```python
from build123d import *

# Parameters (mm, degrees)
SKETCH1_W            = 23
SKETCH1_H            = 12
BOSS_EXTRUDE1_DEPTH  = 18
SKETCH2_W            = 32
SKETCH2_H            = 12
BOSS_EXTRUDE2_DEPTH  = 2.5
SKETCH3_W            = 23
SKETCH3_H            = 12
BOSS_EXTRUDE3_DEPTH  = 4
BOSS_EXTRUDE4_DEPTH  = 4.5
FILLET1_R            = 1
FILLET2_R            = 0.5
CUT_EXTRUDE2_DEPTH   = 21.5
SKETCH5_R            = 2.5
BOSS_EXTRUDE5_DEPTH  = 3
SKETCH6_R            = 1
CUT_EXTRUDE1_DEPTH   = 3
BOSS_EXTRUDE11_DEPTH = 2
FILLET3_R            = 0.5


with BuildPart() as part:
    # Sketch1 → Boss-Extrude1 (new body)
    with BuildSketch(Plane(origin=(0, 0, 0), x_dir=(1, 0, 0), z_dir=(0, 1, 0))):
        Rectangle(SKETCH1_W, SKETCH1_H)
    extrude(amount=BOSS_EXTRUDE1_DEPTH)

    # Sketch2 → Boss-Extrude2 (add)
    with BuildSketch(Plane(origin=(0, 18, 0), x_dir=(1, 0, 0), z_dir=(0, 1, 0))):
        Rectangle(SKETCH2_W, SKETCH2_H)
    extrude(amount=BOSS_EXTRUDE2_DEPTH)

    # Sketch3 → Boss-Extrude3 (add)
    with BuildSketch(Plane(origin=(0, 20.5, 0), x_dir=(1, 0, 0), z_dir=(0, 1, 0))):
        Rectangle(SKETCH3_W, SKETCH3_H)
    extrude(amount=BOSS_EXTRUDE3_DEPTH)

    # Sketch4 → Boss-Extrude4 (add)
    with BuildSketch(Plane(origin=(0, 24.5, 0), x_dir=(1, 0, 0), z_dir=(0, 1, 0))):
        with BuildLine():
            Line((-0.802804538, 3), (0.303847577, 3))
            ThreePointArc((0.303847577, 3), (11.5, 0), (0.303847577, -3))
            Line((0.303847577, -3), (-0.802804538, -3))
            ThreePointArc((-0.802804538, -3), (-3.802804538, 0), (-0.802804538, 3))
        make_face()
    extrude(amount=BOSS_EXTRUDE4_DEPTH)

    # Fillet1
    fillet1_edges = [part.edges().sort_by_distance(p)[0] for p in [
        (11.5, 22.5, 6),
        (11.5, 22.5, -6),
        (-11.5, 22.5, -6),
        (-11.5, 22.5, 6),
        (11.5, 9, 6),
        (-11.5, 9, 6),
        (-11.5, 9, -6),
        (11.5, 9, -6),
    ]]
    fillet(fillet1_edges, radius=FILLET1_R)

    # Fillet2
    fillet2_edges = [part.edges().sort_by_distance(p)[0] for p in [
        (16, 19.25, 6),
        (16, 19.25, -6),
        (-16, 19.25, -6),
        (-16, 19.25, 6),
    ]]
    fillet(fillet2_edges, radius=FILLET2_R)

    # Sketch7 → Cut-Extrude2 (cut, through all)
    with BuildSketch(Plane(origin=(0, 20.5, 0), x_dir=(1, 0, 0), z_dir=(0, 1, 0))):
        with BuildLine():
            Line((14.420576737, 0.3), (16, 0.3))
            Line((16, 0.3), (16, -0.3))
            Line((16, -0.3), (14.420576737, -0.3))
            ThreePointArc((14.420576737, -0.3), (12.53177403, 0), (14.420576737, 0.3))
        make_face()
    cut_extrude2 = extrude(amount=-CUT_EXTRUDE2_DEPTH, mode=Mode.SUBTRACT)

    # Mirror1: Cut-Extrude2 across plane
    add(cut_extrude2.mirror(Plane(origin=(0, 0, 0), x_dir=(0, 0, 1), z_dir=(1, 0, 0))), mode=Mode.SUBTRACT)

    # Sketch5 → Boss-Extrude5 (add)
    with BuildSketch(Plane(origin=(0, 29, 0), x_dir=(1, 0, 0), z_dir=(0, 1, 0))):
        with Locations((5.5, 0)):
            Circle(SKETCH5_R)
    extrude(amount=BOSS_EXTRUDE5_DEPTH)

    # Sketch6 → Cut-Extrude1 (cut)
    with BuildSketch(Plane(origin=(0, 32, 0), x_dir=(1, 0, 0), z_dir=(0, 1, 0))):
        with Locations((5.5, 0)):
            Circle(SKETCH6_R)
    extrude(amount=-CUT_EXTRUDE1_DEPTH, mode=Mode.SUBTRACT)

    # Sketch8 → Boss-Extrude11 (add)
    with BuildSketch(Plane(origin=(11.5, 0, 0), x_dir=(0, 0, -1), z_dir=(1, 0, 0))):
        with BuildLine():
            Line((-0.539222972, 6.176789317), (-0.474627778, 6.176789317))
            ThreePointArc((-0.474627778, 6.176789317), (-0.006925375, 6.5), (0.460777028, 6.176789317))
            Line((0.460777028, 6.176789317), (0.525372222, 6.176789317))
            ThreePointArc((0.525372222, 6.176789317), (1.493074625, 6), (0.525372222, 5.823210683))
            Line((0.525372222, 5.823210683), (0.460777028, 5.823210683))
            ThreePointArc((0.460777028, 5.823210683), (-0.006925375, 5.5), (-0.474627778, 5.823210683))
            Line((-0.474627778, 5.823210683), (-0.539222972, 5.823210683))
            ThreePointArc((-0.539222972, 5.823210683), (-1.506925375, 6), (-0.539222972, 6.176789317))
        make_face()
    extrude(amount=BOSS_EXTRUDE11_DEPTH)

    # Fillet3
    fillet3_edges = [part.edges().sort_by_distance(p)[0] for p in [
        (-3.802804538, 29, 0),
        (-0.249478481, 29, 3),
        (11.5, 29, 0),
        (-0.249478481, 29, -3),
    ]]
    fillet(fillet3_edges, radius=FILLET3_R)


solid = part.part
```
Could you check a few things on this model? Use its own coordinates, in mm. A direction names the side the tool comes from. Give positions to 0.01 mm unless a question says otherwise; leave off trailing zeros. Loops run counter-clockwise (first coordinate to the right, second up) from the corner with the lowest first, then second, coordinate; pieces in that order, holes last. Notation, with made-up numbers: (36, 73) -> (58, 73) arc R20 cw to (58, 84) -> close; hole circle Ø5 at (-21, 35). An arc over 180 degrees is marked (long way). Put each result on its own line as item: value.
(1) Imagine slicing it at C-C on x = -8. Write out the boundary of the cut face in (y, z).
Computed:
outline: (0, -6) -> (24.5, -6) -> (24.5, 6) -> (0, 6) -> close
(2) For faces 5 (the face through (11.5, 22, 0)), 6 (the face through (10, 24.5, -5)), 7 (the face through (-11.215, 22.528, -5.699)), which set-ups out of +Z, -Z, +X, -X, +Y, -Y let a thin tool reach every point of the face, with its end or its side?
Computed:
face 5: +Z, -Z, +X, +Y
face 6: -Z, +X, +Y
face 7: -Z, -X, +Y
(3) Imagine slicing it at B-B on y = 7. Write out the boundary of the cut face in (x, z), plus the area to 3 significant figures.
Computed:
outline: (-11.5, -5) arc R1 ccw to (-10.5, -6) -> (10.5, -6) arc R1 ccw to (11.5, -5) -> (11.5, 5) arc R1 ccw to (10.5, 6) -> (-10.5, 6) arc R1 ccw to (-11.5, 5) -> close
area: 275 mm^2
(4) Imagine slicing it at A-A on x = -13.5. Write out the boundary of the cut face in (y, z), plus the area to 3 significant figures.
Computed:
outline: (18, -6) -> (20.5, -6) -> (20.5, -0.97) -> (18, -0.97) -> close; (18, 0.97) -> (20.5, 0.97) -> (20.5, 6) -> (18, 6) -> close
area: 25.2 mm^2
(5) Please list where these lines run through material, in increasing order: probe 1 along Z at (x, y) = (-13.5, 19.2); probe 2 along X at (y, z) = (30.3, 0); probe 3 along X at (y, z) = (18.7, 0). Write a range as [from, to].
Computed:
probe 1: [-6, -0.97], [0.97, 6]
probe 2: [3, 4.5], [6.5, 8]
probe 3: [-12.53, 12.53]
(6) Thinking about a two-plate mould opening in X: for faces 1 (the face through (-11.5, 9, 0)), 2 (the face through (-15, 19, -0.3)), 3 (the face through (-12.533, 19.268, 0.038)), 4 (the face through (5, 29, 0)), which applies, pulls with the +X half, pulls with the -X half, needs draft (parallel to the pull), parting line crosses it, or undercut?
Computed:
face 1: pulls with the -X half
face 2: needs draft
face 3: undercut
face 4: undercut
(7) I'm going to push flat-ended pins straight in: pin 1 Ø3 at (x, z) = (-13.5, 2.5) entering from +Y; pin 2 Ø3 at (x, z) = (-1.5, -2.5) entering from +Y; pin 3 Ø2 at (y, z) = (28.5, -1) entering from -X. Where does each tip first touch, or does it pass through?
Computed:
pin 1: y = 20.5
pin 2: y = 29
pin 3: x = -3.8
